Autodesk Fusion 360 part; units mm, degrees
sketch "스케치1" plane through (0, 0, 0) normal (0, 0, 1) x (1, 0, 0)
  line L0 (0, 0) -> (60, 0)
  line L1 (60, 0) -> (60, 30)
  line L2 (60, 30) -> (0, 30)
  line L3 (0, 30) -> (0, 0)
  dimension "d1" = 60
  dimension "d2" = 30
extrude "돌출1" add sketch "스케치1" along normal blind 2
sketch "스케치2" plane through (0, 0, 2) normal (0, 0, 1) x (-1, 0, 0)
  circle A0 centre (-53.75, -8.1) radius 1.1
  circle A1 centre (-25.95, -8.1) radius 1.1
  circle A2 centre (-15, -8.1) radius 5
  line L0 (0, 0) -> (-60, 0)
  line L1 (-51.35, -2) -> (-51.35, -14.2)
  line L2 (-51.35, -14.2) -> (-28.35, -14.2)
  line L3 (-28.35, -14.2) -> (-28.35, -2)
  line L4 (-51.35, -2) -> (-28.35, -2)
  dimension "d5" = 2.2
  dimension "d6" = 27.8
  dimension "d8" = 8.1
  dimension "d9" = 10
  dimension "d11" = 15
  dimension "d28" = 25.95
  dimension "d91" = 23
  dimension "d93" = 2.4
  dimension "d94" = 2
  dimension "d95" = 12.2
extrude "돌출2" cut sketch "스케치2" against normal blind 2 contours A0 | A1 | L1 L2 L3 L4
extrude "돌출3" add sketch "스케치2" along normal blind 9 contours A2
sketch "스케치4" plane through (0, 0, 11) normal (0, 0, 1) x (-1, 0, 0)
  circle A0 centre (-15, -8.1) radius 2.3
  circle A1 centre (-15, -8.1) radius 5
  dimension "d34" = 4.6
extrude "돌출5" add sketch "스케치4" along normal blind 2 contours A0
sketch "스케치5" plane through (0, 0, 2) normal (0, 0, 1) x (-1, 0, 0)
  line L0 (0, -30) -> (0, 0)
  line L1 (0, 0) -> (0, -30)
  line L2 (-60, -30) -> (0, -30)
  line L3 (-60, -30) -> (-60, 0)
  line L4 (0, 0) -> (-60, 0)
  line L5 (-60, 0) -> (-54, 0)
  line L6 (-54, -28) -> (-6, -28)
  line L7 (-2, -24) -> (-2, -6)
  line L8 (-6, 0) -> (0, 0)
  line L9 (-58, -24) -> (-58, -6)
  line L10 (-2, -24) -> (-6, -24)
  line L11 (-6, -24) -> (-6, -28)
  line L12 (-54, -28) -> (-54, -24)
  line L13 (-54, -24) -> (-58, -24)
  line L14 (-2, -6) -> (-6, -6)
  line L15 (0, 0) -> (-60, 0)
  line L16 (-6, -6) -> (-6, 0)
  line L17 (-58, -6) -> (-54, -6)
  line L18 (-54, -6) -> (-54, 0)
  point P0 (0, -30)
  point P1 (-60, -30)
  point P2 (-60, 0)
  dimension "d38" = 2
  dimension "d39" = 2
  dimension "d42" = 2
  dimension "d43" = 6
  dimension "d44" = 6
  dimension "d45" = 6
  dimension "d46" = 6
  dimension "d47" = 6
extrude "돌출6" add sketch "스케치5" along normal blind 12 contours L0 L1 L2 L3 L4 L5 L6 L7 L8 L9 L10 L11 L12 L13 L14 L15 L16 L17 L18
sketch "스케치6" plane through (0, 0, 14) normal (0, 0, 1) x (-1, 0, 0)
  circle A0 centre (-3, -27) radius 0.95
  circle A1 centre (-3, -3) radius 0.95
  circle A2 centre (-57, -27) radius 0.95
  circle A3 centre (-57, -3) radius 0.95
  dimension "d48" = 1.9
  dimension "d49" = 3
  dimension "d51" = 3
  dimension "d52" = 24
  dimension "d53" = 54
extrude "돌출7" cut sketch "스케치6" against normal blind 5
fillet "필렛1" radius 3 8 edges at (60, 0, 7) (0, 0, 7) (60, 30, 7) (0, 30, 7) (54, 24, 8) (6, 24, 8) (54, 6, 8) (6, 6, 8)
fillet "필렛1" radius 3 2 edges at (54, 0, 8) (6, 0, 8)
sketch "스케치9" plane through (0, 30, 0) normal (0, 1, 0) x (-1, 0, 0)
  circle A0 centre (-50, 8) radius 1.5
  circle A1 centre (-30, 8) radius 1.5
  circle A2 centre (-10, 8) radius 1.5
  circle A3 centre (-40, 8) radius 1.5
  circle A4 centre (-20, 8) radius 1.5
  dimension "d74" = 3
  dimension "d75" = 8
  dimension "d80" = 10
  dimension "d81" = 10
  dimension "d82" = 10
  dimension "d83" = 10
  dimension "d84" = 10
extrude "돌출10" cut sketch "스케치9" against normal blind 2
Here's how the part is built. I have some questions about the finished solid (model axes, mm). A direction names the side the tool comes from. Coordinates: 2 decimals unless noted, no trailing zeros. Write each loop counter-clockwise with the first axis right and the second up, starting at its lowest first coordinate (ties: lowest second). Pieces come first, ordered by that corner, then holes.
1) Which directions (+Z, -Z, +X, -X, +Y, -Y) give clear straight access to the entire face, cutting with the end or side of a thin tool? Please do faces 1 (the face through (30, 0, 1)), 2 (the face through (21.5, 29.01, 8.07)), 3 (the face through (54.86, 24.9, 8.08)), 4 (the face through (28.35, 8, 1)), 5 (the face through (31.5, 29.01, 8.07)).
Filled in:
face 1: +Z, -Z, +X, -X, -Y
face 2: +Y
face 3: +Z
face 4: +Z, -Z
face 5: +Y, -Y
2) If we section it at A-A (x = 40): List the corners of the cut face in (y, z) for me, plus the area to 3 significant figures.
Filled in:
outline: (0, 0) - (2, 0) - (2, 2) - (0, 2) - close; (14.2, 0) - (30, 0) - (30, 6.5) - (28, 6.5) - (28, 2) - (14.2, 2) - close; (28, 9.5) - (30, 9.5) - (30, 14) - (28, 14) - close
area: 53.6 mm2
3) I'm going to push flat-ended pins straight in: pin 1 (0.5 mm diameter, centred on y = 27.5, z = 11, fed in from +X); pin 2 (2.5 mm diameter, centred on x = 10, z = 8, fed in from -Y); pin 3 (4 mm diameter, centred on x = 31, y = 20, fed in from +Z). Where does each tip first touch, or does it pass through?
Filled in:
pin 1: stops at x = 59.99
pin 2: stops at y = 4.79
pin 3: stops at z = 2
4) If we section it at D-D (y = 22.25): List the corners of the cut face in (x, z) for me.
Filled in:
outline: (0, 0) - (60, 0) - (60, 14) - (58, 14) - (58, 2) - (2, 2) - (2, 14) - (0, 14) - close
5) If I drill on line 1 (X direction, y = 3, z = 10); line 2 (Y direction, x = 57, z = 11); line 3 (X direction, y = 22.25, z = 7.25), over which ranges is the centre line in solid material (lowest first)?
Filled in:
line 1: x = 0 to 2.05, 3.95 to 6, 54 to 56.05, 57.95 to 60
line 2: y = 0 to 2.05, 3.95 to 6, 24 to 26.05, 27.95 to 30
line 3: x = 0 to 2, 58 to 60
6) Thinking about a two-plate mould opening in Y: for faces 6 (the face through (5.1, 0.86, 8.08)), 7 (the face through (57.75, 27.58, 11.54)), 8 (the face through (0.9, 29.14, 7.1)), 9 (the face through (60, 15, 7)), which applies, +Y half, -Y half, draft (parallel to the pull), parting line (faces both ways), or undercut?
Filled in:
face 6: -Y half
face 7: undercut
face 8: +Y half
face 9: draft
7) If we section it at C-C (y = 8.1): List the corners of the cut face in (x, z) for me.
Filled in:
outline: (0, 0) - (24.85, 0) - (24.85, 2) - (20, 2) - (20, 11) - (17.3, 11) - (17.3, 13) - (12.7, 13) - (12.7, 11) - (10, 11) - (10, 2) - (2, 2) - (2, 14) - (0, 14) - close; (27.05, 0) - (28.35, 0) - (28.35, 2) - (27.05, 2) - close; (51.35, 0) - (52.65, 0) - (52.65, 2) - (51.35, 2) - close; (54.85, 0) - (60, 0) - (60, 14) - (58, 14) - (58, 2) - (54.85, 2) - close
